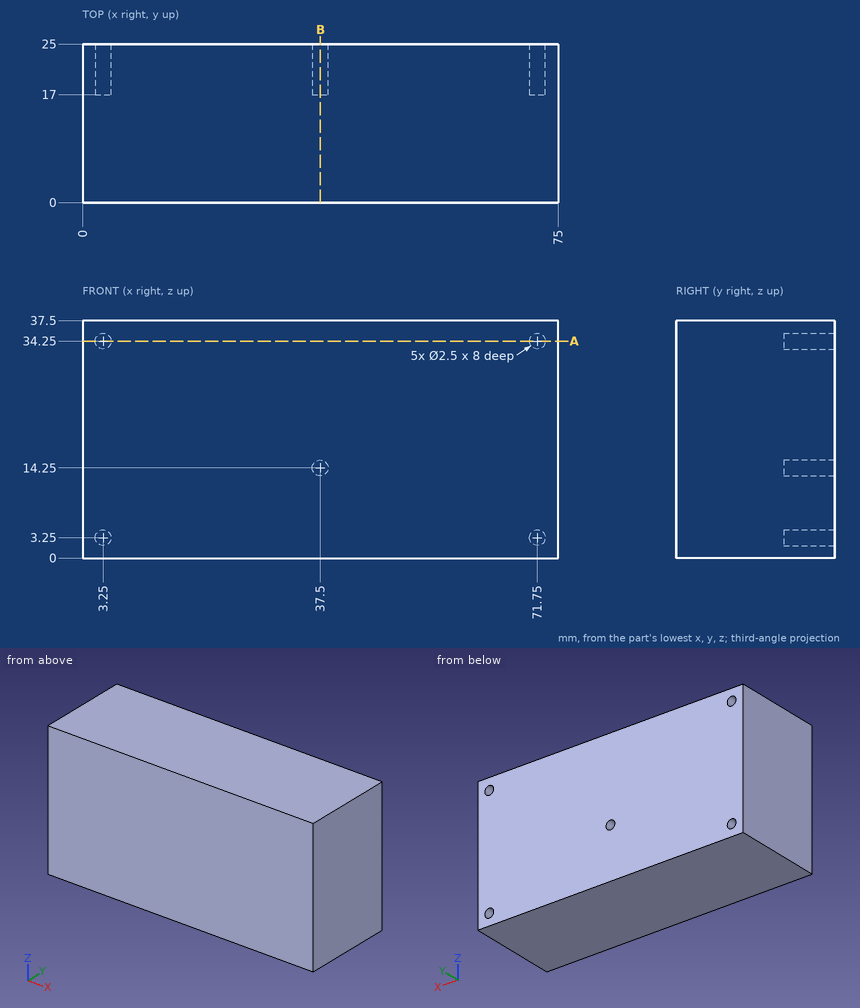
Geometry check sheet. Reference: drawing and pictorial views, mm from the part's lowest x, y, z. Give positions to 0.01 mm unless a question says otherwise; leave off trailing zeros. Write each loop counter-clockwise with the first axis right and the second up, starting at its lowest first coordinate (ties: lowest second). Pieces come first, ordered by that corner, then holes.
Item 1: Cross-section at A-A (z = 34.25). Enter the section's corners in (x, y), and give its area (4 significant figures).
Item 2: Cross-section at B-B (x = 37.5). Enter the section's corners in (y, z).
Item 3: Scan lines: L1, parallel to Z at x = 71.75, y = 20.25; L2, parallel to Z at x = 37.5, y = 21.75. Record each from-to range of solid material in increasing order.
Item 4: Gauge pin test, flat end, axial feed: pin 1 (1.2 mm diameter, centred on x = 71.5, z = 34.5, fed in from +Y). Record the tip position at first contact, or that the pin passes through.
Report:
1. outline: (0, 0) - (75, 0) - (75, 25) - (73, 25) - (73, 17) - (70.5, 17) - (70.5, 25) - (4.5, 25) - (4.5, 17) - (2, 17) - (2, 25) - (0, 25) - close
1. area: 1,835 mm2
2. outline: (0, 0) - (25, 0) - (25, 13) - (17, 13) - (17, 15.5) - (25, 15.5) - (25, 37.5) - (0, 37.5) - close
3. L1: z = 0 to 2, 4.5 to 33, 35.5 to 37.5
3. L2: z = 0 to 13, 15.5 to 37.5
4. pin 1: stops at y = 17
